Source: CAD feature listing. Evaluate the final solid. Frame: model axes, mm. Face numbers are marked on the shaded views. A direction names the side the tool comes from. Give positions to 0.01 mm unless a question says otherwise; leave off trailing zeros. Order: outer loops, then holes, each group sorted by start corner. A loop starts at its lowest first (then second) coordinate and runs counter-clockwise, first axis right, second up. Notation, with made-up numbers: M 15.5,25.5 L 40.5,25.5 A28 cw 40.5,60.5 Z; hole C 84.25,-34.5 d10. An arc over 180 degrees is marked long. One line per question, with ' | ' between items. Start each with the question number.
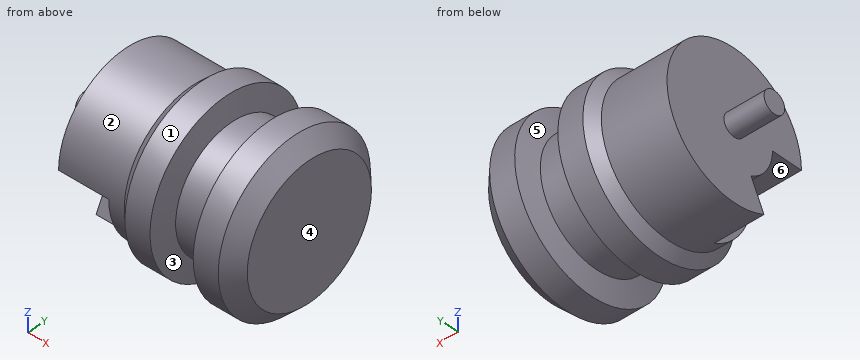
from build123d import *

# Parameters (mm, degrees)
CHAMFER1_SIZE            = 0.75
BOSS_EXTRUDE1_DEPTH      = 3
BOSS_EXTRUDE1_DEPTH_BACK = 1
SKETCH2_R                = 3.6
SKETCH3_R                = 0.55
BOSS_EXTRUDE2_DEPTH      = 2
CUT_EXTRUDE1_DEPTH       = 2.5


with BuildPart() as part:
    # Sketch1 → Revolve1 (revolve)
    with BuildSketch(Plane(origin=(0, 0, 0), x_dir=(1, 0, 0), z_dir=(0, 1, 0)), mode=Mode.PRIVATE) as revolve1_sk:
        Polygon((-4.15, 4.075), (-6.15, 4.075), (-6.15, 0), (0, 0), (0, 4.075), (-2, 4.075), (-2.275, 3), (-3.875, 3), align=None)
    revolve(revolve1_sk.sketch.rotate(Axis((-23.01300908, 0, 0), (1, 0, 0)), 180), axis=Axis((-23.01300908, 0, 0), (1, 0, 0)))

    # Chamfer1
    chamfer1_edges = [part.edges().sort_by_distance(p)[0] for p in [
        (-6.15, 0, -4.075),
        (0, 0, -4.075),
    ]]
    chamfer(chamfer1_edges, length=CHAMFER1_SIZE)

    # Sketch2 → Boss-Extrude1 (add, two sides: drawn at the far end of the back side and taken through both)
    with BuildSketch(Plane.ZY.offset(6.15).offset(-BOSS_EXTRUDE1_DEPTH_BACK)):
        Circle(SKETCH2_R)
    extrude(amount=BOSS_EXTRUDE1_DEPTH + BOSS_EXTRUDE1_DEPTH_BACK)

    # Sketch3 → Boss-Extrude2 (add)
    with BuildSketch(Plane.ZY.offset(9.15)):
        Circle(SKETCH3_R)
    extrude(amount=BOSS_EXTRUDE2_DEPTH)

    # Sketch4 → Cut-Extrude1 (cut)
    with BuildSketch(Plane.ZY.offset(9.15)):
        with BuildLine():
            Line((0, -3.6), (0, -2.05))
            ThreePointArc((0, -2.05), (-1.081944444, -1.741234108), (-1.837969336, -0.907947531))
            Line((-1.837969336, -0.907947531), (-3.227653469, -1.594444444))
            ThreePointArc((-3.227653469, -1.594444444), (-1.9, -3.05777697), (0, -3.6))
        make_face()
    extrude(amount=-CUT_EXTRUDE1_DEPTH, mode=Mode.SUBTRACT)


solid = part.part
Item 1: Cut plane D-D on x = -5. Return the cut outline in (y, z) (3 decimals), and give its area (3 significant figures).
Item 2: Cut plane C-C on x = -7.5. Return the cut outline in (y, z), and give its area (3 significant figures).
Item 3: Line query: line 1 (X direction, y = -2, z = 0.25); line 2 (X direction, y = 3, z = 1.5); line 3 (X direction, y = 0.25, z = -3.25). Output: solid intervals per line, ascending.
Item 4: Cut plane A-A on y = 0. Return the cut outline in (x, z) (3 decimals).
Item 5: Mould query, pull axis X, two halves, no side actions, for the marked faces 4, 5 and 6. Classes: pulls with the +X half, pulls with the -X half, needs draft (parallel to the pull), parting line crosses it, or undercut.
Item 6: Cut plane B-B on x = -10. Return the cut outline in (y, z), and give its area (3 significant figures).
Item 7: Reachability of the marked faces 1, 2 and 3 from +Z, -Z, +X, -X, +Y, -Y: full face, straight path, thin tool, end or side. Return the list, or none.
Item 8: Pin query (flat end, axial travel): pin 1 Ø0.5 at (x, y) = (-8.5, -3) entering from -Z; pin 2 Ø0.8 at (y, z) = (-3, -2) entering from -X; pin 3 Ø1 at (y, z) = (3, -1) entering from -X; pin 4 Ø3.5 at (y, z) = (0, 1) entering from -X. Return the tip coordinate at first contact, or that it passes through.
Results are:
1) outline: C 0,0 d8.15 | area: 52.2 mm2
2) outline: M -3.6,0 L -2.05,0 A2.05 ccw -0.91,-1.84 L -1.59,-3.23 A3.6 ccw long Z | area: 35.8 mm2
3) line 1: x = -9.15 to 0 | line 2: x = -9.15 to -3.97, -2.18 to -0.03 | line 3: x = -9.15 to -3.94, -2.21 to 0
4) outline: M -11.15,-0.55 L -9.15,-0.55 L -9.15,-3.6 L -5.875,-3.6 L -5.4,-4.075 L -4.15,-4.075 L -3.875,-3 L -2.275,-3 L -2,-4.075 L -0.75,-4.075 L 0,-3.325 L 0,3.325 L -0.75,4.075 L -2,4.075 L -2.275,3 L -3.875,3 L -4.15,4.075 L -5.4,4.075 L -5.875,3.6 L -9.15,3.6 L -9.15,0.55 L -11.15,0.55 Z
5) face 4: pulls with the +X half | face 5: undercut | face 6: needs draft
6) outline: C 0,0 d1.1 | area: 0.950 mm2
7) face 1: +X, -X | face 2: -X | face 3: none
8) pin 1: stops at z = 0 | pin 2: stops at x = -6.65 | pin 3: stops at x = -9.15 | pin 4: stops at x = -11.15
